from build123d import *

# Parameters (mm, degrees)
F0_W      = 152.4
F0_H      = 127
F1_DEPTH  = 6.35
F2_R      = 2.25
F3_DEPTH  = 6.351
F4_R      = 2.5
F5_DEPTH  = 25.4
F6_R      = 4.75
F7_DEPTH  = 3
F8_R      = 2.2479
F9_DEPTH  = 6.351
F10_W     = 3.175
F10_H     = 9.42
F10_W_2   = 149.225
F10_H_2   = 117.58
F11_DEPTH = 6.351
F12_R     = 3.17499
F13_R     = 3.571875
F14_DEPTH = 2.54


# Not quite as in the source:
# - a fillet or chamfer is up to 0.001 mm smaller than in the source, because OpenCascade refuses the exact size


with BuildPart() as f1:
    # F0 (on Top) → F1 (new body)
    with BuildSketch(Plane.XY):
        with Locations((76.2, 63.5)):
            Rectangle(F0_W, F0_H)
    extrude(amount=F1_DEPTH)

    # F2 (on face) → F3 (cut, through all)
    with BuildSketch(Plane.XY.offset(6.35)):
        with Locations((15.3375, 120.65)):
            Circle(F2_R)
        with Locations((140.2375, 120.65)):
            Circle(F2_R)
        with Locations((77.7875, 16.75)):
            Circle(F2_R)
    extrude(amount=-F3_DEPTH, mode=Mode.SUBTRACT)

    # F4 (on face) → F5 (cut)
    with BuildSketch(Plane(origin=(0, 0, 0), x_dir=(1, 0, 0), z_dir=(0, 0, -1))):
        with Locations((45.7875, -67.575)):
            Circle(F4_R)
        with Locations((109.7875, -67.575)):
            Circle(F4_R)
    extrude(amount=-F5_DEPTH, mode=Mode.SUBTRACT)

    # F6 (on face) → F7 (cut)
    with BuildSketch(Plane.XY.offset(6.35)):
        with Locations((45.7875, 67.575)):
            Circle(F6_R)
        with Locations((109.7875, 67.575)):
            Circle(F6_R)
    extrude(amount=-F7_DEPTH, mode=Mode.SUBTRACT)

    # F8 (on face) → F9 (cut, through all)
    with BuildSketch(Plane.XY.offset(6.35)):
        with Locations((146.05, 86.625)):
            Circle(F8_R)
        with Locations((146.05, 48.525)):
            Circle(F8_R)
        with Locations((9.525, 48.525)):
            Circle(F8_R)
        with Locations((9.525, 86.625)):
            Circle(F8_R)
        with Locations((45.7875, 104.405)):
            Circle(F8_R)
        with Locations((109.2875, 104.405)):
            Circle(F8_R)
        with Locations((45.7875, 30.745)):
            Circle(F8_R)
        with Locations((109.2875, 30.745)):
            Circle(F8_R)
    extrude(amount=-F9_DEPTH, mode=Mode.SUBTRACT)

    # F10 (on face) → F11 (cut, through all)
    with BuildSketch(Plane.XY.offset(6.35)):
        with Locations((1.5875, 4.71)):
            Rectangle(F10_W, F10_H)
        with Locations((77.7875, 4.71)):
            Rectangle(F10_W_2, F10_H)
        with Locations((1.5875, 68.21)):
            Rectangle(F10_W, F10_H_2)
    extrude(amount=-F11_DEPTH, mode=Mode.SUBTRACT)

    # F12 (radius 3.175 in the source; OpenCascade refuses exactly that, so slightly less here)
    f12_edges = [f1.edges().sort_by_distance(p)[0] for p in [
        (3.175, 68.21, 6.35),
        (77.7875, 9.42, 6.35),
        (152.4, 68.21, 6.35),
        (77.7875, 127, 6.35),
        (77.7875, 127, 0),
        (3.175, 68.21, 0),
        (77.7875, 9.42, 0),
        (152.4, 68.21, 0),
    ]]
    fillet(f12_edges, radius=F12_R)

    # F13 (on face) → F14 (cut)
    with BuildSketch(Plane.XY):
        with Locations((45.7875, 30.745)):
            Circle(F13_R)
        with Locations((109.2875, 30.745)):
            Circle(F13_R)
        with Locations((9.525, 48.525)):
            Circle(F13_R)
        with Locations((9.525, 86.625)):
            Circle(F13_R)
        with Locations((45.7875, 104.405)):
            Circle(F13_R)
        with Locations((109.2875, 104.405)):
            Circle(F13_R)
        with Locations((146.05, 86.625)):
            Circle(F13_R)
        with Locations((146.05, 48.525)):
            Circle(F13_R)
    extrude(amount=F14_DEPTH, mode=Mode.SUBTRACT)


solid = f1.part
Verification items for the finished model (mm, model axes). A direction names the side the tool comes from. Coordinates: 2 decimals unless noted, no trailing zeros. Use CSV: the item, a comma, the result in double quotes.
Q1. Thickness scan on line 1 along X through (y, z) = (68, 2.5); line 2 along X through (y, z) = (85.5, 3.25); line 3 along Z through (x, y) = (107.5, 65). Record the ranges inside material, lowest first. Write a range as [from, to].
Computed values:
line 1,"[3.25, 43.32], [48.25, 107.32], [112.25, 152.33]"
line 2,"[3.18, 7.58], [11.47, 144.1], [148, 152.4]"
line 3,"[0, 3.35]"
Q2. Go/stop test with flat-tipped pins: P1, Ø3.5, axis at x = 110.5, y = 30, coming from the -Z side; P2, Ø8, axis at x = 109.79, y = 67.58, coming from the +Z side. Record where each tip stops, or that it passes through.
Computed values:
P1,"z = 2.54"
P2,"z = 3.35"
Q3. Section check A-A, the plane y = 120.65. State how many separate pieces and enclosed holes the cut face has, and give its area (3 significant figures).
Computed values:
separate pieces,"3"
enclosed holes,"0"
area,"882 mm²"
Q4. Mould release check, pull along X, two halves, no side actions. Record for faces 1 (the flat face through (46, 28, 2.54)), 2 (the cylindrical face through (78.83, 126.09, 0.95)): pulls with the +X half, pulls with the -X half, needs draft (parallel to the pull), parting line crosses it, or undercut.
Computed values:
face 1,"undercut"
face 2,"needs draft"
Q5. Set-up check for faces 3 (the cylindrical face through (8.75, 83.14, 1.25)), 4 (the flat face through (112, 66, 3.35)), 5 (the cylindrical face through (76.74, 10.37, 5.44)): record each of +Z, -Z, +X, -X, +Y, -Y from which the full face is reachable in a straight line by a thin tool's end or side.
Computed values:
face 3,"-Z"
face 4,"+Z"
face 5,"+Z, +X, -X, -Y"
